Answer from the drawing. Dimensions are ordinates in mm from the lowest x, y and z of the part. A direction names the side the tool comes from. Coordinates: 2 decimals unless noted, no trailing zeros. Order: outer loops, then holes, each group sorted by start corner. A loop starts at its lowest first (then second) coordinate and runs counter-clockwise, first axis right, second up. Notation, with made-up numbers: M -6.75,88 L 12.25,88 A21 cw 12.25,126 Z; hole C 4,75.5 d3. An arc over 180 degrees is marked long. Use a Markdown table: item, result.
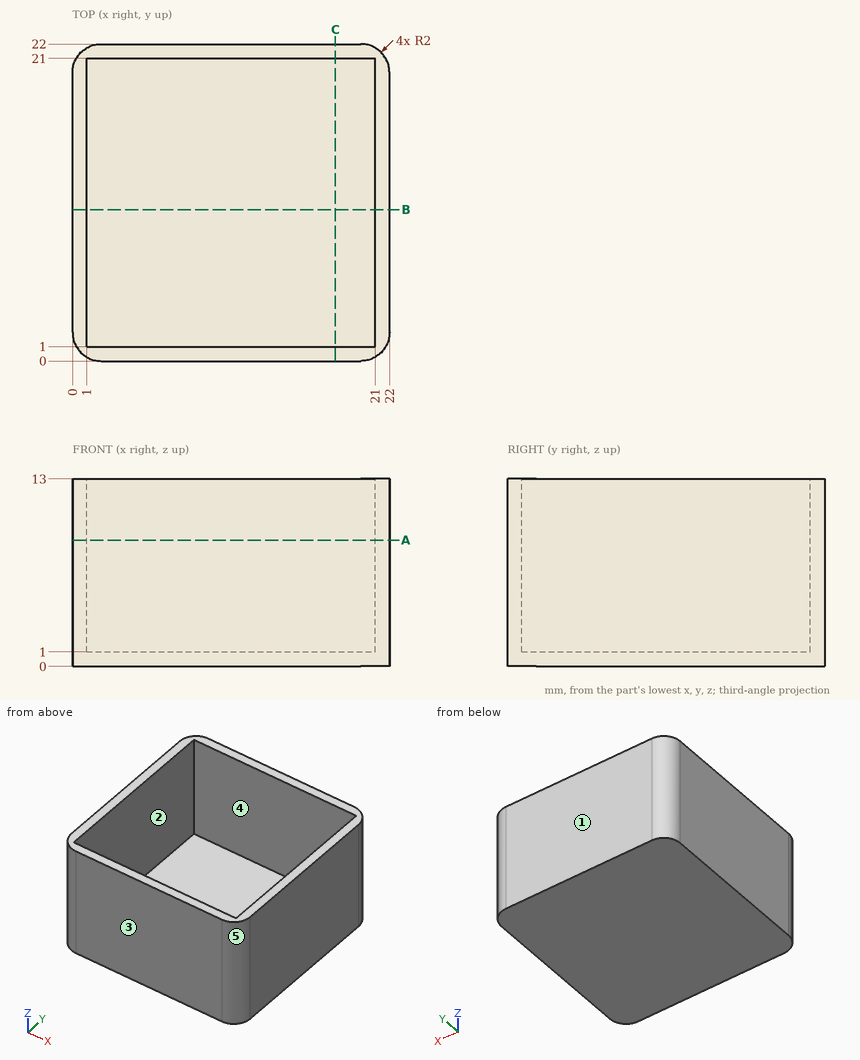
(1) Determine the mould class of the marked faces 1, 2 and 3 for opening direction Y: pulls with the +Y half, pulls with the -Y half, needs draft (parallel to the pull), parting line crosses it, or undercut.
Conclusion:
| item | result |
|---|---|
| face 1 | pulls with the +Y half |
| face 2 | undercut |
| face 3 | pulls with the -Y half |
(2) A cutting plane is placed at B-B (y = 10.5). Determine the outline of the cut face in (x, z), then the cut area to 3 significant figures.
Conclusion:
| item | result |
|---|---|
| outline | M 0,0 L 22,0 L 22,13 L 21,13 L 21,1 L 1,1 L 1,13 L 0,13 Z |
| area | 46.0 mm2 |
(3) Which of the six approach directions +Z, -Z, +X, -X, +Y, -Y give full straight-line access (tool end or side, diameter ignored) to the marked faces 4 and 5?
Conclusion:
| item | result |
|---|---|
| face 4 | +Z |
| face 5 | +Z, -Z, +X, -Y |
(4) Straight lines are drawn through the part: L1, parallel to Y at x = 10.75, z = 11.5; L2, parallel to Z at x = 4.5, y = 5. For each, find the intervals that lie inside material, in ascending order.
Conclusion:
| item | result |
|---|---|
| L1 | 0 to 1, 21 to 22 |
| L2 | 0 to 1 |
(5) A cutting plane is placed at A-A (z = 8.75). Determine the outline of the cut face in (x, y), then the cut area to 3 significant figures.
Conclusion:
| item | result |
|---|---|
| outline | M 0,2 A2 ccw 2,0 L 20,0 A2 ccw 22,2 L 22,20 A2 ccw 20,22 L 2,22 A2 ccw 0,20 Z; hole M 1,1 L 21,1 L 21,21 L 1,21 Z |
| area | 80.6 mm2 |
